Autodesk Inventor part; units mm, degrees
ref_plane "YZ Plane" through (0, 0, 0) normal (1, 0, 0) x (0, 1, 0)
ref_plane "XZ Plane" through (0, 0, 0) normal (0, 1, 0) x (-1, 0, 0)
ref_plane "XY Plane" through (0, 0, 0) normal (0, 0, 1) x (1, 0, 0)
sketch "スケッチ1" plane through (0, 0, 0) normal (0, 0, 1) x (1, 0, 0)
  line L0 (0, 0) -> (40, 0)
  line L1 (40, 0) -> (40, 25)
  line L2 (40, 25) -> (0, 25)
  line L3 (0, 25) -> (0, 0)
  dimension "d0" = 40
  dimension "d1" = 25
extrude "押し出し1" add sketch "スケッチ1" along normal blind 6
sketch "スケッチ2" plane through (0, 0, 6) normal (0, 0, 1) x (1, 0, 0)
  circle A0 centre (20, 12.5) radius 9.5
  line L0 (0, 0) -> (40, 0)
  line L1 (0, 25) -> (0, 0)
  dimension "d4" = 19
  dimension "d5" = 12.5
  dimension "d6" = 20
extrude "押し出し2" cut sketch "スケッチ2" against normal blind 6
sketch "スケッチ3" plane through (0, 0, 6) normal (0, 0, 1) x (1, 0, 0)
  circle A0 centre (5, 12.5) radius 1.6
  circle A1 centre (35, 12.5) radius 1.6
  line L0 (0, 25) -> (0, 0)
  line L1 (0, 0) -> (40, 0)
  line L2 (40, 0) -> (40, 25)
  dimension "d9" = 3.2
  dimension "d10" = 3.2
  dimension "d11" = 5
  dimension "d12" = 12.5
  dimension "d13" = 5
  dimension "d14" = 12.5
hole "穴1" at (5, 12.5, 6) at (35, 12.5, 6) direction (0, 0, -1) diameter 3.2 depth 6
equation "\"BendRadius\" = Thickness"
equation "\"BendReliefWidth\" = Thickness"
equation "\"BendReliefDepth\" = 0.5 * Thickness"
equation "\"CornerReliefSize\" = 4 * Thickness"
equation "\"MinimumRemnant\" = 2 * Thickness"
equation "\"TransitionRadius\" = BendRadius"
equation "\"JacobiRadiusSize\" = BendRadius"
equation "\"GapSize\" = Thickness"
properties part number "nhk46"
Check sheet for the modelled part. Datum: model origin and axes. Units: mm. Round coordinates to 2 decimals unless told otherwise and drop trailing zeros. Order: outer loops, then holes, each group sorted by start corner. A loop starts at its lowest first (then second) coordinate and runs counter-clockwise, first axis right, second up. Notation, with made-up numbers: M -21.5,20 L -12.5,20 A16 cw -12.5,29 Z; hole C 57.25,36.25 d3. An arc over 180 degrees is marked long. One line per item, written item: value. Start each with the question number.
1. Section check C-C on y = 18.5. Enter the section's corners in (x, z).
2. Section check A-A on x = 5. Enter the section's corners in (y, z).
3. Release check for a two-part mould opening along Y. For faces 1 (the cylindrical face through (35.97, 13.77, 2.96)), 2 (the flat face through (10.8, 15.5, 0)), 3 (the cylindrical face through (4.93, 14.1, 2.96)), 4 (the flat face through (20, 25, 3)) record: released by +Y, released by -Y, zero draft, split by the parting line, or undercut.
4. Section check B-B on z = 4.45. Enter the section's corners in (x, y).
5. Gauge pin test, flat end, axial feed: P1, Ø4, axis at x = 5, y = 12.5, coming from the +Z side. Record the tip position at first contact, or that the pin passes through.
6. Scan lines: line 1 along Y through (x, z) = (35, 2.8); line 2 along Y through (x, z) = (16, 5.5); line 3 along X through (y, z) = (7.5, 4.8). Record each from-to range of solid material in increasing order.
Results found:
1. outline: M 0,0 L 12.63,0 L 12.63,6 L 0,6 Z; M 27.37,0 L 40,0 L 40,6 L 27.37,6 Z
2. outline: M 0,0 L 10.9,0 L 10.9,6 L 0,6 Z; M 14.1,0 L 25,0 L 25,6 L 14.1,6 Z
3. face 1: undercut
3. face 2: zero draft
3. face 3: undercut
3. face 4: released by +Y
4. outline: M 0,0 L 40,0 L 40,25 L 0,25 Z; hole C 5,12.5 d3.2; hole C 20,12.5 d19; hole C 35,12.5 d3.2
5. P1: z = 6
6. line 1: 0 to 10.9, 14.1 to 25
6. line 2: 0 to 3.88, 21.12 to 25
6. line 3: 0 to 11.92, 28.08 to 40
